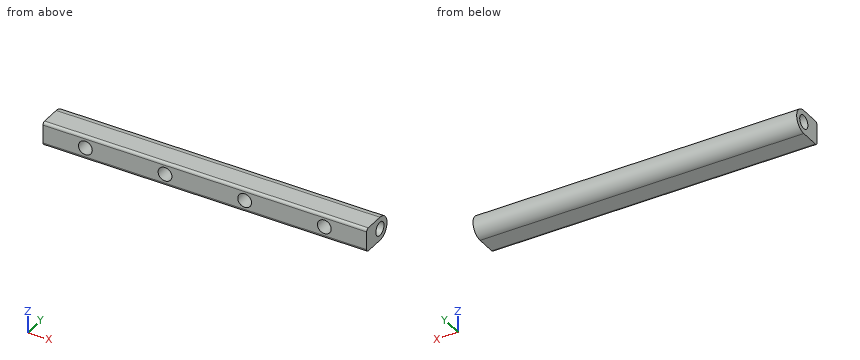
from build123d import *

# Parameters (mm, degrees)
SKETCH1_R                      = 6.35
EXTRUDE1_DEPTH                 = 152.4
EXTRUDE1_DEPTH_BACK            = 152.4
F_13_0_13_DIAMETER_HOLE1_D     = 13
F_13_0_13_DIAMETER_HOLE1_DEPTH = 20.6365
F_13_0_13_DIAMETER_HOLE1_TIP   = 3.905594024


with BuildPart() as part:
    # Sketch1 → Extrude1 (new body, two sides)
    with BuildSketch(Plane(origin=(0, 0, 0), x_dir=(0, 0, -1), z_dir=(1, 0, 0))) as extrude1_sk:
        with BuildLine():
            Line((-11.1125, 0), (-11.1125, -18.0975))
            ThreePointArc((-11.1125, -18.0975), (-10.368551224, -19.893551224), (-8.5725, -20.6375))
            Line((-8.5725, -20.6375), (8.5725, -20.6375))
            ThreePointArc((8.5725, -20.6375), (10.368551224, -19.893551224), (11.1125, -18.0975))
            Line((11.1125, -18.0975), (11.1125, 0))
            ThreePointArc((11.1125, 0), (0, 11.1125), (-11.1125, 0))
        make_face()
        Circle(SKETCH1_R, mode=Mode.SUBTRACT)
    extrude(amount=EXTRUDE1_DEPTH)
    extrude(extrude1_sk.sketch, amount=-EXTRUDE1_DEPTH_BACK)

    # 13.0 _13_ Diameter Hole1
    with Locations(Plane(origin=(-112.5, -20.6375, 0), x_dir=(0, 0, -1), z_dir=(0, -1, 0))):
        with Locations((0, 0), (0, 75), (0, 150), (0, 225)):
            Hole(F_13_0_13_DIAMETER_HOLE1_D / 2, depth=F_13_0_13_DIAMETER_HOLE1_DEPTH)
            with Locations((0, 0, -(F_13_0_13_DIAMETER_HOLE1_DEPTH + F_13_0_13_DIAMETER_HOLE1_TIP / 2))):  # 118° drill point
                Cone(0, F_13_0_13_DIAMETER_HOLE1_D / 2, F_13_0_13_DIAMETER_HOLE1_TIP, mode=Mode.SUBTRACT)


solid = part.part
Work out the finished part from the listing and answer in its coordinate system (mm). Round coordinates to 2 decimals unless told otherwise and drop trailing zeros. Loops run counter-clockwise (first coordinate to the right, second up) from the corner with the lowest first, then second, coordinate; pieces in that order, holes last. Notation, with made-up numbers: (-16.5, 37.25) - (-12.5, 37.25) arc R23 cw to (-12.5, 49.25) - close; hole circle Ø1 at (60.5, 86.25). An arc over 180 degrees is marked (long way). Use one line per item in the form item = value. Start each with the question number.
(1) Consider line 1 (X direction, y = -14.75, z = 0); line 2 (Y direction, x = 105, z = -0.75); line 3 (X direction, y = -12, z = -2.75). Determine where each line is inside the solid, lowest interval first.
(2) Flat-ended cylindrical pins translate along their axes: P1, Ø8, axis at y = 0, z = -5.5, coming from the -X side; P2, Ø8, axis at x = -112.5, z = 0, coming from the -Y side; P3, Ø7.5, axis at y = 0, z = 0, coming from the +X side; P4, Ø3, axis at x = -18.5, z = -5, coming from the +Y side. Find the tip coordinate at first contact, or state that the pin passes through.
(3) Find section C-C on y = -9.5. Determine the outline of the cut face in (x, z), and give its area (3 significant figures).
(4) Find section B-B on z = 0. Determine the outline of the cut face in (x, y), and give its area (3 significant figures).
Answer list:
q1.line_1 = -152.4 to -119, -106 to -44, -31 to 31, 44 to 106, 119 to 152.4
q1.line_2 = -20.64 to -6.31, 6.31 to 11.09
q1.line_3 = -152.4 to -118.39, -106.61 to -43.39, -31.61 to 31.61, 43.39 to 106.61, 118.39 to 152.4
q2.P1 = -152.4
q2.P2 = 4.93
q2.P3 = through
q2.P4 = 10.55
q3.outline = (-152.4, -11.11) - (152.4, -11.11) - (152.4, 11.11) - (-152.4, 11.11) - close; hole circle Ø13 at (-112.5, 0); hole circle Ø13 at (-37.5, 0); hole circle Ø13 at (37.5, 0); hole circle Ø13 at (112.5, 0)
q3.area = 6,240 mm^2
q4.outline = (-152.4, -20.64) - (-119, -20.64) - (-119, -6.35) - (-152.4, -6.35) - close; (-152.4, 6.35) - (152.4, 6.35) - (152.4, 11.11) - (-152.4, 11.11) - close; (-106, -20.64) - (-44, -20.64) - (-44, -6.35) - (-106, -6.35) - close; (-31, -20.64) - (31, -20.64) - (31, -6.35) - (-31, -6.35) - close; (44, -20.64) - (106, -20.64) - (106, -6.35) - (44, -6.35) - close; (119, -20.64) - (152.4, -20.64) - (152.4, -6.35) - (119, -6.35) - close
q4.area = 5,060 mm^2
